Geometry: final body of the model. Coordinates: model frame, mm. A direction names the side the tool comes from. Round coordinates to 2 decimals unless told otherwise and drop trailing zeros. Loops run counter-clockwise (first coordinate to the right, second up) from the corner with the lowest first, then second, coordinate; pieces in that order, holes last. Notation, with made-up numbers: (81, 23.25) - (107, 23.25) arc R14 cw to (107, 28.25) - close; hole circle Ø9 at (46, 60). An arc over 180 degrees is marked (long way). Answer as CSV lines item,"result".
Autodesk Inventor part; units mm, degrees
ref_plane "YZ Plane" through (0, 0, 0) normal (1, 0, 0) x (0, 1, 0)
ref_plane "XZ Plane" through (0, 0, 0) normal (0, 1, 0) x (-1, 0, 0)
ref_plane "XY Plane" through (0, 0, 0) normal (0, 0, 1) x (1, 0, 0)
sketch "스케치1" plane through (0, 0, 0) normal (0, 0, 1) x (1, 0, 0)
  line L0 (0, 0) -> (-35, 60.6218)
  line L1 (-35, 60.6218) -> (-70, 0)
  line L2 (-70, 0) -> (0, 0)
  line L3 (-61.3397, 5) -> (-35, 50.6218)
  line L4 (-37.8868, 55.6218) -> (-8.6603, 5)
  line L5 (-8.6603, 5) -> (-67.1132, 5)
  line L6 (0, 0) -> (8.6603, 5)
  line L7 (-2.5, 4.3301) -> (6.1603, 9.3301)
  line L8 (6.1603, 9.3301) -> (8.6603, 5)
  line L9 (6.1603, 9.3301) -> (6.1603, 14.3301)
  line L10 (6.1603, 14.3301) -> (8.6603, 14.3301)
  line L11 (8.6603, 5) -> (8.6603, 14.3301)
  line L12 (-35, 60.6218) -> (-35, 0) construction
  line L13 (-70, 0) -> (-78.6603, 5)
  line L14 (-75.7735, 10) -> (-78.6603, 5)
  line L15 (-75.7735, 14.3301) -> (-78.6603, 14.3301)
  line L16 (-78.6603, 5) -> (-78.6603, 14.3301)
  line L17 (-67.1132, 5) -> (-75.7735, 10)
  line L18 (-75.7735, 10) -> (-75.7735, 14.3301)
  line L19 (-70, 0) -> (-78.6603, -5)
  line L20 (-75.7735, -10) -> (-78.6603, -5)
  line L21 (-78.6603, -5) -> (-78.6603, -14.3301)
  line L22 (-73.6603, -14.3301) -> (-78.6603, -14.3301)
  line L23 (-58.453, 0) -> (-75.7735, -10)
  line L24 (-73.6603, -8.7799) -> (-73.6603, -14.3301)
  line L25 (-73.6603, -14.3301) -> (-68.6603, -17.2169)
  line L26 (-68.6603, -17.2169) -> (-68.6603, -20.1036)
  line L27 (-78.6603, -14.3301) -> (-68.6603, -20.1036)
  point P0 (-76.1603, 9.3301)
  point P1 (-76.1603, 14.3301)
  point P2 (-67.1132, -5)
  point P3 (-76.1603, -9.3301)
  point P4 (-76.1603, -14.3301)
  point P5 (-75.7735, -14.3301)
  dimension "d0" = 60
  dimension "d1" = 60
  dimension "d2" = 70
  dimension "d3" = 5
  dimension "d6" = 90
  dimension "d7" = 5
  dimension "d8" = 10
  dimension "d9" = 5
  dimension "d11" = 5
  dimension "d12" = 120
  dimension "d13" = 5
extrude "돌출1" add sketch "스케치1" along normal mid plane 40 contours L2 L1 L5 L4 L0 | L0 L7 L8 L6 | L23 L20 L19 L2 | L8 L9 L10 L11 | L13 L14 L17 L1 | L24 L22 L21 L20 L23 | L16 L15 L18 L14 | L25 L26 L27 L22
fillet "모깎기1" radius 2 18 edges at (-75.7735, 10, 0) (-67.1132, 5, 0) (-2.5, 4.3301, 0) (-8.6603, 5, 0) (6.1603, 9.3301, 0) (-37.8868, 55.6218, 0) (-35, 60.6218, 0) (-75.7735, 14.3301, 0) (6.1603, 14.3301, 0) (-78.6603, 5, 0) (-70, 0, 0) (0, 0, 0) (8.6603, 5, 0) (-78.6603, -5, 0) (-58.453, 0, 0) (-73.6603, -8.7799, 0) (-73.6603, -14.3301, 0) (-68.6603, -17.2169, 0)
(1) Section A-A (x = -19). Output: boundary loops of the cut face in (y, z), and give its area (3 significant figures).
Findings below:
outline,"(0, -20) - (5, -20) - (5, 20) - (0, 20) - close; (22.91, -20) - (32.91, -20) - (32.91, 20) - (22.91, 20) - close"
area,"600 mm2"
(2) Pin query (flat end, axial travel): P1, Ø1, axis at y = -12, z = -8, coming from the +X side; P2, Ø3, axis at x = -53.5, z = 5, coming from the +Y side; P3, Ø1, axis at y = 23.5, z = -14, coming from the +X side. Return the tip coordinate at first contact, or that it passes through.
Findings below:
P1,"x = -73.66"
P2,"y = 5"
P3,"x = -13.28"
(3) Section B-B (x = -51). Output: boundary loops of the cut face in (y, z), and give its area (3 significant figures).
Findings below:
outline,"(0, -20) - (5, -20) - (5, 20) - (0, 20) - close"
area,"200 mm2"
(4) Draft query along Y for faces 6 (the face through (-30, 0, 0)), 7 (the face through (-38, 2, -20)), 8 (the face through (-71.18, -15.76, -0.28)). Return one class per face: pulls with the +Y half, pulls with the -Y half, needs draft (parallel to the pull), parting line crosses it, or undercut.
Findings below:
face 6,"pulls with the -Y half"
face 7,"needs draft"
face 8,"undercut"
(5) Material intervals for line 1 along X through (y, z) = (10.5, 12); line 2 along Y through (x, z) = (-36.5, 11.5); line 3 along Y through (x, z) = (-44, -5), sorted ascending.
Findings below:
line 1,"-78.66 to -75.66, -11.84 to -6.06, 6.16 to 8.66"
line 2,"0 to 5, 53.22 to 57.94"
line 3,"0 to 5"
(6) Access query for faces 1 (the face through (6.76, 13.76, 0.28)), 2 (the face through (-39, 5, 0)), 3 (the face through (-75.3, -3.06, -0.28)), 4 (the face through (8.66, 10, 0)), 5 (the face through (-65.69, -4.18, -0.28)). Directions: +Z, -Z, +X, -X, +Y, -Y. A direction counts if a zero-diameter tool reaches every point of the face in a straight line with its end or side. Return the directions, or none.
Findings below:
face 1,"+Z, -Z, +Y"
face 2,"+Z, -Z"
face 3,"+Z, -Z, -X"
face 4,"+Z, -Z, +X, +Y, -Y"
face 5,"+Z, -Z, +X"
(7) Section C-C (y = 27). Output: boundary loops of the cut face in (x, z).
Findings below:
outline,"(-21.36, -20) - (-15.59, -20) - (-15.59, 20) - (-21.36, 20) - close"
